```python
from build123d import *

# Parameters (mm, degrees)
SKETCH1_R                = 1.55
BOSS_EXTRUDE1_DEPTH      = 1.75
SKETCH2_R                = 1.55
BOSS_EXTRUDE2_DEPTH      = 2.7
BOSS_EXTRUDE3_DEPTH      = 30.5
BOSS_EXTRUDE3_DEPTH_BACK = 30.5
CUT_EXTRUDE1_DEPTH       = 14.7
CHAMFER2_SIZE            = 3
FILLET2_R                = 1


with BuildPart() as part:
    # Sketch1 → Boss-Extrude1 (new, symmetric)
    # profile 1 of 3: a face of its own
    with BuildSketch(Plane(origin=(0, 0, 0), x_dir=(1, 0, 0), z_dir=(0, 1, 0))):
        Polygon((-10.5, -31.5), (-30.5, -11.5), (-30.5, 31.5), (30.5, 31.5), (30.5, -11.5), (10.5, -31.5), align=None)
    # profile 2 of 3: a face of its own
    with BuildSketch(Plane(origin=(0, 0, 0), x_dir=(1, 0, 0), z_dir=(0, 1, 0))):
        with BuildLine():
            Line((20.5, 31.5), (30.5, 31.5))
            Line((30.5, 31.5), (30.5, 37.5))
            ThreePointArc((30.5, 37.5), (29.328427125, 40.328427125), (26.5, 41.5))
            Line((26.5, 41.5), (20.5, 41.5))
            Line((20.5, 41.5), (20.5, 31.5))
        make_face()
        with Locations(Location((25.5, 36.5, 0), (0, 0, 270))):
            Circle(SKETCH1_R, mode=Mode.SUBTRACT)
    # profile 3 of 3: a face of its own
    with BuildSketch(Plane(origin=(0, 0, 0), x_dir=(1, 0, 0), z_dir=(0, 1, 0))):
        with BuildLine():
            Line((-30.5, 31.5), (-20.5, 31.5))
            Line((-20.5, 31.5), (-20.5, 41.5))
            Line((-20.5, 41.5), (-26.5, 41.5))
            ThreePointArc((-26.5, 41.5), (-29.328427125, 40.328427125), (-30.5, 37.5))
            Line((-30.5, 37.5), (-30.5, 31.5))
        make_face()
        with Locations(Location((-25.5, 36.5, 0), (0, 0, 270))):
            Circle(SKETCH1_R, mode=Mode.SUBTRACT)
    extrude(amount=BOSS_EXTRUDE1_DEPTH, both=True)

    # Sketch2 → Boss-Extrude2 (add)
    # profile 1 of 3: a face of its own
    with BuildSketch(Plane(origin=(0, 1.75, 0), x_dir=(1, 0, 0), z_dir=(0, 1, 0))):
        with BuildLine():
            Line((-20.5, 31.5), (-20.5, 41.5))
            Line((-20.5, 41.5), (-26.5, 41.5))
            ThreePointArc((-26.5, 41.5), (-29.328427125, 40.328427125), (-30.5, 37.5))
            Line((-30.5, 37.5), (-30.5, 31.5))
            Line((-30.5, 31.5), (-20.5, 31.5))
        make_face()
        with Locations(Location((-25.5, 36.5, 0), (0, 0, 270))):
            Circle(SKETCH2_R, mode=Mode.SUBTRACT)
    # profile 2 of 3: a face of its own
    with BuildSketch(Plane(origin=(0, 1.75, 0), x_dir=(1, 0, 0), z_dir=(0, 1, 0))):
        Polygon((20.5, 31.5), (-20.5, 31.5), (-30.5, 31.5), (-30.5, 28.5), (30.5, 28.5), (30.5, 31.5), align=None)
    # profile 3 of 3: a face of its own
    with BuildSketch(Plane(origin=(0, 1.75, 0), x_dir=(1, 0, 0), z_dir=(0, 1, 0))):
        with BuildLine():
            Line((20.5, 41.5), (20.5, 31.5))
            Line((20.5, 31.5), (30.5, 31.5))
            Line((30.5, 31.5), (30.5, 37.5))
            ThreePointArc((30.5, 37.5), (29.328427125, 40.328427125), (26.5, 41.5))
            Line((26.5, 41.5), (20.5, 41.5))
        make_face()
        with Locations(Location((25.5, 36.5, 0), (0, 0, 270))):
            Circle(SKETCH2_R, mode=Mode.SUBTRACT)
    extrude(amount=BOSS_EXTRUDE2_DEPTH)

    # Sketch3 → Boss-Extrude3 (add, two sides: drawn at the far end of the back side and taken through both)
    with BuildSketch(Plane(origin=(0, 0, 0), x_dir=(0, 0, -1), z_dir=(1, 0, 0)).offset(-BOSS_EXTRUDE3_DEPTH_BACK)):
        Polygon((28.5, 1.75), (-31.5, 1.75), (28.5, 16.45), align=None)
    extrude(amount=BOSS_EXTRUDE3_DEPTH + BOSS_EXTRUDE3_DEPTH_BACK)

    # Sketch4 → Cut-Extrude1 (cut)
    with BuildSketch(Plane(origin=(0, 16.45, 0), x_dir=(-1, 0, 0), z_dir=(0, -1, 0))):
        Polygon((26.5, -15.5), (26.5, 24.5), (1.5, 24.5), (1.5, -31.5), (10.5, -31.5), align=None)
        Polygon((-26.5, -15.5), (-10.5, -31.5), (-1.5, -31.5), (-1.5, 24.5), (-26.5, 24.5), align=None)
        Polygon((26.5, -31.5), (26.5, -15.5), (10.5, -31.5), align=None)
        Polygon((30.5, -11.5), (26.5, -15.5), (26.5, -31.5), (30.5, -31.5), align=None)
        Polygon((-26.5, -15.5), (-26.5, -31.5), (-10.5, -31.5), align=None)
        Polygon((-30.5, -31.5), (-26.5, -31.5), (-26.5, -15.5), (-30.5, -11.5), align=None)
    extrude(amount=CUT_EXTRUDE1_DEPTH, mode=Mode.SUBTRACT)

    # Chamfer2
    chamfer2_edges = [part.edges().sort_by_distance(p)[0] for p in [
        (28.5, 6.16, 13.5),
        (14, 15.47, -24.5),
        (-14, 15.47, -24.5),
        (-28.5, 6.16, 13.5),
        (-30.5, 11.55, -8.5),
        (30.5, 11.55, -8.5),
    ]]
    chamfer(chamfer2_edges, length=CHAMFER2_SIZE)

    # Fillet2
    fillet2_edges = [part.edges().sort_by_distance(p)[0] for p in [
        (1.5, 8.966943345, 2.043088387),
        (-1.5, 8.966943345, 2.043088387),
    ]]
    fillet(fillet2_edges, radius=FILLET2_R)


solid = part.part
```
CAD build for the part. Positions are in the model's coordinates, mm. A direction names the side the tool comes from. Coordinates: 2 decimals unless noted, no trailing zeros. Order: outer loops, then holes, each group sorted by start corner. A loop starts at its lowest first (then second) coordinate and runs counter-clockwise, first axis right, second up. Notation, with made-up numbers: (44.5, -6.75) -> (98.5, -6.75) arc R30 cw to (98.5, 26.25) -> close; hole circle Ø7 at (44, 10). An arc over 180 degrees is marked (long way). Use one line per item in the form item = value. Start each with the question number.
1) Band-saw the part on C-C on y = 0.25. Give the cut face in (x, z), then the cut area to 3 significant figures.
2) Drop flat-ended pins along their axis: pin 1 (5 mm diameter, centred on x = -5, y = 0, fed in from -Z); pin 2 (1 mm diameter, centred on x = -8.5, y = 9, fed in from -Z); pin 3 (6 mm diameter, centred on x = 8, y = 12.5, fed in from +Z); pin 4 (6.5 mm diameter, centred on x = -7.5, z = -35.5, fed in from +Y). Give the stop position or say it passes through.
3) Band-saw the part on A-A on x = 25.5. Give the cut face in (y, z), then the cut area to 3 significant figures.
4) Band-saw the part on D-D on x = -15.5. Give the cut face in (y, z), then the cut area to 3 significant figures.
5) Pull direction X, two halves, no side cores. Call faces 4 (the cylindrical face through (-1.2, 8.59, 2.39)), 5 (the flat face through (-30.5, 4, -13)), 6 (the flat face through (-7, 4.45, -31)): +X half, -X half, draft (parallel to the pull), parting line (faces both ways), or undercut.
6) Tool access for faces 1 (the flat face through (-20.5, 1, -36)), 2 (the cylindrical face through (-24.19, 1.31, -35.67)), 3 (the flat face through (-13, 1.75, 3)): list every direction of +Z, -Z, +X, -X, +Y, -Y with a clear straight run to the whole face (end or side of a thin tool).
7) Band-saw the part on B-B on z = -36.5. Give the cut face in (x, y), then the cut area to 3 significant figures.
8) Drill centre lines: L1, parallel to X at y = 8.75, z = -24; L2, parallel to X at y = 1.5, z = -36.5; L3, parallel to Z at x = 11.5, y = 2. Where is each one in solid material? Low to high. Write a range as [from, to].
Entries:
q1.outline = (-30.5, -37.5) arc R4 ccw to (-26.5, -41.5) -> (-20.5, -41.5) -> (-20.5, -31.5) -> (20.5, -31.5) -> (20.5, -41.5) -> (26.5, -41.5) arc R4 ccw to (30.5, -37.5) -> (30.5, 11.5) -> (10.5, 31.5) -> (-10.5, 31.5) -> (-30.5, 11.5) -> close; hole circle Ø3.1 at (-25.5, -36.5); hole circle Ø3.1 at (25.5, -36.5)
q1.area = 3,620 mm2
q2.pin_1 = -31.5
q2.pin_2 = -28.5
q2.pin_3 = -24.5
q2.pin_4 = through
q3.outline = (-1.75, -41.5) -> (4.45, -41.5) -> (4.45, -38.05) -> (-1.75, -38.05) -> close; (-1.75, -34.95) -> (4.45, -34.95) -> (4.45, -28.5) -> (16.45, -28.5) -> (16.18, -27.41) -> (12.47, -24.5) -> (1.75, -24.5) -> (1.75, 16.5) -> (-1.75, 16.5) -> close
q3.area = 271 mm2
q4.outline = (-1.75, -31.5) -> (4.45, -31.5) -> (4.45, -28.5) -> (16.45, -28.5) -> (16.18, -27.41) -> (12.47, -24.5) -> (1.75, -24.5) -> (1.75, 26.5) -> (-1.75, 26.5) -> close
q4.area = 264 mm2
q5.face_4 = undercut
q5.face_5 = -X half
q5.face_6 = draft
q6.face_1 = -Z, +Y, -Y
q6.face_2 = +Y, -Y
q6.face_3 = +Z, +Y
q7.outline = (-30.5, -1.75) -> (-27.05, -1.75) -> (-27.05, 4.45) -> (-30.5, 4.45) -> close; (-23.95, -1.75) -> (-20.5, -1.75) -> (-20.5, 4.45) -> (-23.95, 4.45) -> close; (20.5, -1.75) -> (23.95, -1.75) -> (23.95, 4.45) -> (20.5, 4.45) -> close; (27.05, -1.75) -> (30.5, -1.75) -> (30.5, 4.45) -> (27.05, 4.45) -> close
q7.area = 85.6 mm2
q8.L1 = [-30.5, -26.5], [-1.5, 1.5], [26.5, 30.5]
q8.L2 = [-30.5, -27.05], [-23.95, -20.5], [20.5, 23.95], [27.05, 30.5]
q8.L3 = [-31.5, -24.5]
